Autodesk Inventor part; units mm, degrees
ref_plane "YZ Plane" through (0, 0, 0) normal (1, 0, 0) x (0, 1, 0)
ref_plane "XZ Plane" through (0, 0, 0) normal (0, 1, 0) x (-1, 0, 0)
ref_plane "XY Plane" through (0, 0, 0) normal (0, 0, 1) x (1, 0, 0)
sketch "Sketch1" plane through (0, 0, 0) normal (0, 1, 0) x (-1, 0, 0)
  line L0 (0, 0) -> (-134.9375, 0) construction
  line L1 (0, 4.7625) -> (-134.9375, 4.7625)
  line L2 (-134.9375, -4.7625) -> (0, -4.7625)
  arc A0 (0, -4.7625) -> (0, 4.7625) centre (0, 0) ccw
  arc A1 (-134.9375, 4.7625) -> (-134.9375, -4.7625) centre (-134.9375, 0) ccw
  circle A2 centre (0, 0) radius 2
  circle A3 centre (-134.9375, 0) radius 2
  line L3 (0, 4.7625) -> (-25.4, 4.7625)
  line L4 (-25.4, 4.7625) -> (-25.4, 11.1125)
  line L5 (-25.4, 11.1125) -> (0, 11.1125)
  line L6 (0, 11.1125) -> (0, 4.7625)
  line L7 (-25.4, 7.9375) -> (0, 7.9375) construction
  circle A4 centre (-22.225, 7.9375) radius 1.5
  circle A5 centre (-17.4625, 7.9375) radius 1.5
  circle A6 centre (-12.7, 7.9375) radius 1.5
  circle A7 centre (-7.9375, 7.9375) radius 1.5
  circle A8 centre (-3.175, 7.9375) radius 1.5
  point P0 (-67.4688, 0)
  dimension "d0" = 134.9375
  dimension "d1" = 9.525
  dimension "d2" = 4
  dimension "d3" = 4
  dimension "d6" = 25.4
  dimension "d7" = 6.35
  dimension "d8" = 3
  dimension "d9" = 3.175
  dimension "d12" = 4.7625
extrude "Extrusion1" add sketch "Sketch1" along normal blind 3.175
fillet "Fillet1" radius 3.175 4 edges at (25.4, 1.5875, 4.7625) (25.4, 1.5875, 11.1125) (0, 1.5875, 11.1125) (0, 1.5875, 4.7625)
equation "\"d2\" = d3"
properties part number "Wind Tool"
Check sheet for the modelled part. Datum: model origin and axes. Units: mm. A direction names the side the tool comes from. Round coordinates to 2 decimals unless told otherwise and drop trailing zeros. Order: outer loops, then holes, each group sorted by start corner. A loop starts at its lowest first (then second) coordinate and runs counter-clockwise, first axis right, second up.
(1) Cross-section at C-C, the plane y = 1.5. State how many separate pieces and enclosed holes the cut face has, and give its area (3 significant figures).
(2) Cross-section at D-D, the plane x = 62. Enter the section's corners in (y, z) (1 decimal), and give its area (3 significant figures).
(3) Cross-section at A-A, the plane x = 12.7. Enter the section's corners in (y, z) (1 decimal), and give its area (3 significant figures).
(4) Draft check along Z on faces 3 (the cylindrical face through (139.7, 1.6, -0.1)), 4 (the flat face through (13, 2, 11.112)), 5 (the cylindrical face through (18.96, 1.57, 7.87)). Enter one of: pulls with the +Z half, pulls with the -Z half, needs draft (parallel to the pull), parting line crosses it, or undercut.
(5) Scan lines: probe 1 along X at (y, z) = (0.25, -1.5); probe 2 along Z at (x, y) = (131, 1.6); probe 3 along Z at (x, y) = (12.7, 1.5). Record each from-to range of solid material in increasing order.
(6) Cross-section at B-B, the plane z = 0. Enter the section's corners in (x, y) (1 decimal), and give its area (3 significant figures).
(7) Go/stop test with flat-tipped pins: P1, Ø1.6, axis at x = 63, y = 1, coming from the +Z side; P2, Ø2.5, axis at x = 17.46, z = 7.94, coming from the -Y side. Record where each tip stops, or that it passes through.
(8) Access from +Z, -Z, +X, -X, +Y, -Y to the whole of each face (thin tool, end or side, straight path). Record for faces 1 (the flat face through (81, 2, 4.762)), 2 (the cylindrical face through (3.5, 1.6, 9.4)).
Check sheet entries:
1. separate pieces: 1
1. enclosed holes: 7
1. area: 1,460 mm2
2. outline: (0, -4.8) - (3.2, -4.8) - (3.2, 4.8) - (0, 4.8) - close
2. area: 30.2 mm2
3. outline: (0, -4.8) - (3.2, -4.8) - (3.2, 6.4) - (0, 6.4) - close; (0, 9.4) - (3.2, 9.4) - (3.2, 11.1) - (0, 11.1) - close
3. area: 40.9 mm2
4. face 3: parting line crosses it
4. face 4: pulls with the +Z half
4. face 5: undercut
5. probe 1: x = -4.52 to -1.32, 1.32 to 133.61, 136.26 to 139.46
5. probe 2: z = -4.76 to 4.76
5. probe 3: z = -4.76 to 6.44, 9.44 to 11.11
6. outline: (-4.8, 0) - (-2, 0) - (-2, 3.2) - (-4.8, 3.2) - close; (2, 0) - (132.9, 0) - (132.9, 3.2) - (2, 3.2) - close; (136.9, 0) - (139.7, 0) - (139.7, 3.2) - (136.9, 3.2) - close
6. area: 433 mm2
7. P1: stops at z = 4.76
7. P2: passes through
8. face 1: +Z, +X, +Y, -Y
8. face 2: +Y, -Y
